```python
from build123d import *

# Parameters (mm, degrees)
CROQUIS1_W              = 54
CROQUIS1_H              = 54
SALIENTE_EXTRUIR1_DEPTH = 60
CROQUIS2_R              = 13
CORTAR_EXTRUIR1_DEPTH   = 72.119617547
CROQUIS3_R              = 20
CORTAR_EXTRUIR2_DEPTH   = 14
CORTAR_EXTRUIR3_START   = -12
CROQUIS4_R              = 20
CORTAR_EXTRUIR3_DEPTH   = 12
CROQUIS5_R              = 3.25
CORTAR_EXTRUIR4_DEPTH   = 72.119617547
REDONDEO1_R             = 4
CHAFL_N1_SIZE           = 1


with BuildPart() as part:
    # Croquis1 → Saliente-Extruir1 (new body)
    with BuildSketch(Plane.XY):
        Rectangle(CROQUIS1_W, CROQUIS1_H)
    extrude(amount=SALIENTE_EXTRUIR1_DEPTH)

    # Croquis2 → Cortar-Extruir1 (cut, through all)
    with BuildSketch(Plane.XY.offset(60)):
        Circle(CROQUIS2_R)
    extrude(amount=-CORTAR_EXTRUIR1_DEPTH, mode=Mode.SUBTRACT)

    # Croquis3 → Cortar-Extruir2 (cut)
    with BuildSketch(Plane.XY.offset(60)):
        Circle(CROQUIS3_R)
    extrude(amount=-CORTAR_EXTRUIR2_DEPTH, mode=Mode.SUBTRACT)

    # Croquis4 → Cortar-Extruir3 (cut)
    with BuildSketch(Plane(origin=(0, 0, 0), x_dir=(-1, 0, 0), z_dir=(0, 0, -1)).offset(CORTAR_EXTRUIR3_START)):
        with Locations(Location((0, 0, 0), (0, 0, 180))):
            Circle(CROQUIS4_R)
    extrude(amount=CORTAR_EXTRUIR3_DEPTH, mode=Mode.SUBTRACT)

    # Croquis5 → Cortar-Extruir4 (cut, through all)
    with BuildSketch(Plane.XY.offset(60)):
        with Locations((20, 20)):
            Circle(CROQUIS5_R)
        with Locations((20, -20)):
            Circle(CROQUIS5_R)
        with Locations((-20, -20)):
            Circle(CROQUIS5_R)
        with Locations((-20, 20)):
            Circle(CROQUIS5_R)
    extrude(amount=-CORTAR_EXTRUIR4_DEPTH, mode=Mode.SUBTRACT)

    # Redondeo1
    redondeo1_edges = [part.edges().sort_by_distance(p)[0] for p in [
        (27, -27, 30),
        (-27, -27, 30),
        (-27, 27, 30),
        (27, 27, 30),
    ]]
    fillet(redondeo1_edges, radius=REDONDEO1_R)

    # Chaflán1
    chafl_n1_edges = [part.edges().sort_by_distance(p)[0] for p in [
        (16.75, 20, 60),
        (16.75, -20, 60),
        (-23.25, -20, 60),
        (-23.25, 20, 60),
    ]]
    chamfer(chafl_n1_edges, length=CHAFL_N1_SIZE)


solid = part.part
```
Part model, mm, in its own coordinate system. A direction names the side the tool comes from. Give positions to 0.01 mm unless a question says otherwise; leave off trailing zeros. Order: outer loops, then holes, each group sorted by start corner. A loop starts at its lowest first (then second) coordinate and runs counter-clockwise, first axis right, second up. Notation, with made-up numbers: M 22.5,87.25 L 62.5,87.25 A18 cw 62.5,112.25 Z; hole C -22,36.25 d7. An arc over 180 degrees is marked long. Use a Markdown table: item, result. Add a question column.
(1) Mould opens along X. For faces 1 (the face through (-25.859, 25.797, 30.42)), 2 (the face through (13, 4, 12)), 3 (the face through (-12, 18, 60)) say: +X half, -X half, draft (parallel to the pull), parting line (faces both ways), or undercut.
(2) Drop flat-ended pins along their axis: P1, Ø10.5, axis at x = 20, y = 20, coming from the -Z side; P2, Ø8, axis at x = 12, y = -10, coming from the +Z side; P3, Ø12, axis at x = 7.5, y = 3.5, coming from the -Z side. Give the stop position or say it passes through.
(3) Saw through at D-D, the plane z = 10. Give the cut face in (x, y).
(4) 3-axis set-ups, long thin cutter, end or side, ignore diameter. For faces 4 (the face through (25.797, -25.859, 30.42)), 5 (the face through (-4.336, -19.524, 53.098)), 6 (the face through (-19.98, -0.88, 6.08)): which of +Z, -Z, +X, -X, +Y, -Y reach the whole face in a straight line?
(5) Saw through at A-A, the plane y = 0. Give the cut face in (x, z).
(6) Probe line 1 along Y through (x, z) = (-20, 16); line 2 along Y through (x, z) = (21, 44.5); line 3 along Y through (x, z) = (0, 49). List the from-to ranges inside material, lowest first. Write a range as [from, to].
(7) Saw through at B-B, the plane z = 37. Give the cut face in (x, y).
Answer key:
| question | item | result |
|---|---|---|
| 1 | face 1 | -X half |
| 1 | face 2 | undercut |
| 1 | face 3 | draft |
| 2 | P1 | z = 0 |
| 2 | P2 | z = 46 |
| 2 | P3 | z = 12 |
| 3 | outline | M -27,-23 A4 ccw -23,-27 L 23,-27 A4 ccw 27,-23 L 27,23 A4 ccw 23,27 L -23,27 A4 ccw -27,23 Z; hole C -20,-20 d6.5; hole C -20,20 d6.5; hole C 0,0 d40; hole C 20,-20 d6.5; hole C 20,20 d6.5 |
| 4 | face 4 | +Z, -Z, +X, -Y |
| 4 | face 5 | +Z |
| 4 | face 6 | -Z |
| 5 | outline | M -27,0 L -20,0 L -20,12 L -13,12 L -13,46 L -20,46 L -20,60 L -27,60 Z; M 13,12 L 20,12 L 20,0 L 27,0 L 27,60 L 20,60 L 20,46 L 13,46 Z |
| 6 | line 1 | [-27, -23.25], [-16.75, 16.75], [23.25, 27] |
| 6 | line 2 | [-27, -23.09], [-16.91, 16.91], [23.09, 27] |
| 6 | line 3 | [-27, -20], [20, 27] |
| 7 | outline | M -27,-23 A4 ccw -23,-27 L 23,-27 A4 ccw 27,-23 L 27,23 A4 ccw 23,27 L -23,27 A4 ccw -27,23 Z; hole C -20,-20 d6.5; hole C -20,20 d6.5; hole C 0,0 d26; hole C 20,-20 d6.5; hole C 20,20 d6.5 |
